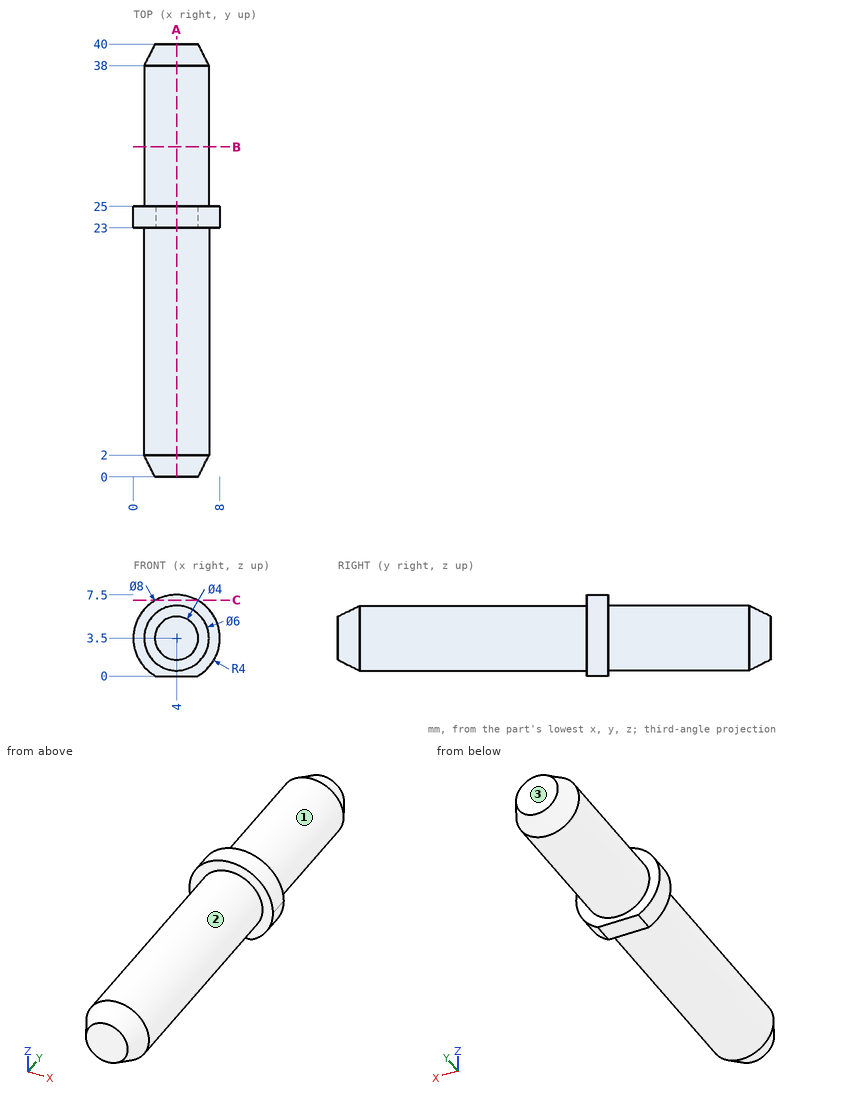
Could you check a few things on this drawing? It's one solid part, dimensions in mm from its lowest x, y, z. A direction names the side the tool comes from. Give positions to 0.01 mm unless a question says otherwise; leave off trailing zeros. Write each loop counter-clockwise with the first axis right and the second up, starting at its lowest first coordinate (ties: lowest second). Pieces come first, ordered by that corner, then holes. Notation, with made-up numbers: (-33, 43) -> (19, 43) arc R23 ccw to (19, 71) -> close; hole circle Ø8 at (11, 4). An arc over 180 degrees is marked (long way). Answer as CSV lines item,"result". Start each with the question number.
(1) Which directions (+Z, -Z, +X, -X, +Y, -Y) give clear straight access to the entire face, cutting with the end or side of a thin tool? Please do the marked faces 1, 2 and 3.
(2) If we section it at A-A, the plane x = 4: Write out the boundary of the cut face in (y, z).
(3) I'm going to push flat-ended pins straight in: pin 1 Ø3 at (x, y) = (6, 7.5) entering from -Z; pin 2 Ø2 at (x, y) = (4, 15.5) entering from +Z; pin 3 Ø2 at (y, z) = (6, 2) entering from +X. Where does each tip first touch, or does it pass through?
(4) Please list where these lines run through material, in increasing order: line 1 (Y direction, x = 4, z = 7); line 2 (X direction, y = 14.5, z = 5.5); line 3 (Z direction, x = 6.75, y = 10.5).
(5) If we section it at C-C, the plane z = 7: Write out the boundary of the cut face in (x, y), and give its area (3 significant figures).
(6) If we section it at B-B, the plane y = 30.5: Write out the boundary of the cut face in (x, z), and give its area (3 significant figures).
Answer list:
1,face 1,"+Y"
1,face 2,"-Y"
1,face 3,"+Z, -Z, +X, -X, +Y"
2,outline,"(0, 1.5) -> (2, 0.5) -> (23, 0.5) -> (23, 0) -> (25, 0) -> (25, 0.5) -> (38, 0.5) -> (40, 1.5) -> (40, 5.5) -> (38, 6.5) -> (25, 6.5) -> (25, 7.5) -> (23, 7.5) -> (23, 6.5) -> (2, 6.5) -> (0, 5.5) -> close"
3,pin 1,"z = 0.54"
3,pin 2,"z = 6.5"
3,pin 3,"x = 6.96"
4,line 1,"23 to 25"
4,line 2,"1.76 to 6.24"
4,line 3,"2.3 to 4.7"
5,outline,"(2.06, 23) -> (5.94, 23) -> (5.94, 25) -> (2.06, 25) -> close"
5,area,"7.75 mm^2"
6,outline,"circle Ø6 at (4, 3.5)"
6,area,"28.3 mm^2"
